Drawing for the job (mm, zero at the part's lowest x, y, z). Round coordinates to 2 decimals unless told otherwise and drop trailing zeros. Order: outer loops, then holes, each group sorted by start corner. A loop starts at its lowest first (then second) coordinate and runs counter-clockwise, first axis right, second up. Notation, with made-up numbers: (55, 75.25) - (112, 75.25) arc R20 cw to (112, 91.25) - close; hole circle Ø11 at (-18.75, 46). An arc over 180 degrees is marked (long way). One line per question, with ' | ' between items. Start each with the question number.
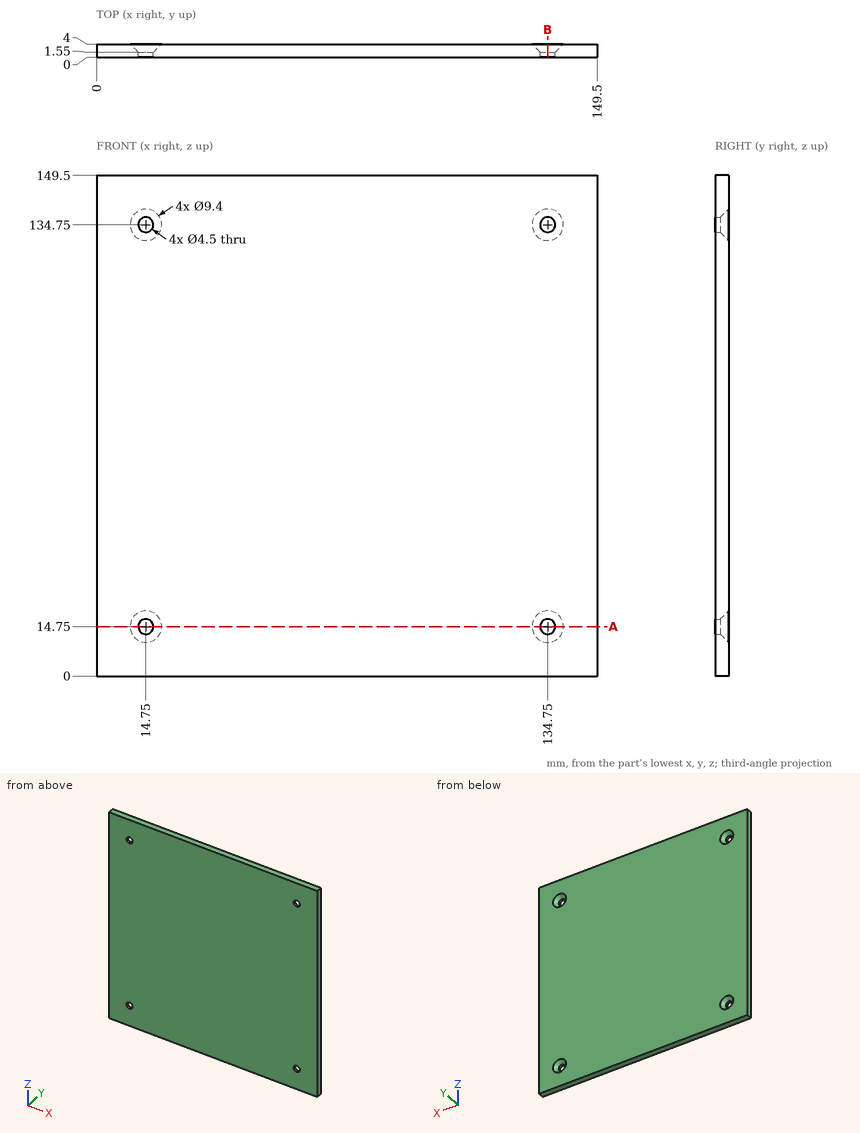
Item 1: Wall check: line 1 along X through (y, z) = (0.9, 134.75); line 2 along Z through (x, y) = (17, 3.1). Give the ranges that are in metal, low to high. Write a range as [from, to].
Item 2: Slice it at B-B (x = 134.75). Write the cut outline in (y, z).
Item 3: Pin check, flat tips, straight feed: pin 1 (3.5 mm diameter, centred on x = 14.75, z = 14.75, fed in from +Y); pin 2 (6 mm diameter, centred on x = 134.75, z = 134.75, fed in from +Y). Stop position of each tip, or through.
Item 4: Slice it at A-A (z = 14.75). Write the cut outline in (x, y), plus the area to 3 significant figures.
A:
1) line 1: [0, 12.5], [17, 132.5], [137, 149.5] | line 2: [0, 11.69], [17.81, 131.69], [137.81, 149.5]
2) outline: (0, 0) - (4, 0) - (4, 10.05) - (1.55, 12.5) - (0, 12.5) - close; (0, 17) - (1.55, 17) - (4, 19.45) - (4, 130.05) - (1.55, 132.5) - (0, 132.5) - close; (0, 137) - (1.55, 137) - (4, 139.45) - (4, 149.5) - (0, 149.5) - close
3) pin 1: through | pin 2: y = 2.3
4) outline: (0, 0) - (12.5, 0) - (12.5, 1.55) - (10.05, 4) - (0, 4) - close; (17, 0) - (132.5, 0) - (132.5, 1.55) - (130.05, 4) - (19.45, 4) - (17, 1.55) - close; (137, 0) - (149.5, 0) - (149.5, 4) - (139.45, 4) - (137, 1.55) - close | area: 550 mm^2
